Verification items for the finished model (mm, model axes). A direction names the side the tool comes from. Give positions to 0.01 mm unless a question says otherwise; leave off trailing zeros. Write each loop counter-clockwise with the first axis right and the second up, starting at its lowest first coordinate (ties: lowest second). Pieces come first, ordered by that corner, then holes. Notation, with made-up numbers: (84, 67) -> (131, 67) arc R26 ccw to (131, 100) -> close; hole circle Ø11 at (18, -14). An arc over 180 degrees is marked (long way). Use one line per item in the form item = value. Start each with the question number.
(1) Section check B-B, the plane x = 16.5. Record the cut outline in (y, z), plus the area to 3 significant figures.
(2) Set-up check for faces 1 (the face through (22, -11, 63.508)), 2 (the face through (21, 0, 34)): record each of +Z, -Z, +X, -X, +Y, -Y from which the full face is reachable in a straight line by a thin tool's end or side.
(3) Section check C-C, the plane y = -14.25. Record the cut outline in (x, z).
(4) Depth check by flat-ended pin: pin 1 Ø16.5 at (x, z) = (28.5, 30) entering from -Y; pin 2 Ø3.5 at (x, y) = (43.5, -12) entering from -Z; pin 3 Ø10.5 at (x, y) = (44.5, -13) entering from +Z. Enter the tip coordinate at first touch or a pass-through.
(5) Release check for a two-part mould opening along X. For faces 3 (the face through (53, -10, 32)), 4 (the face through (47, -10, 65)), 5 (the face through (0, -11, 61)) record: pulls with the +X half, pulls with the -X half, needs draft (parallel to the pull), parting line crosses it, or undercut.
(6) Section check A-A, the plane z = 59. Record the cut outline in (x, y), plus the area to 3 significant figures.
(7) Scan lines: L1, parallel to X at y = -9.5, z = 17.5; L2, parallel to Z at x = 3.5, y = -4.5; L3, parallel to Y at x = 24, z = 47. Record each from-to range of solid material in increasing order.
from build123d import *

# Parameters (mm, degrees)
F2_DEPTH  = 2
F0_W      = 4
F0_H      = 4
F0_H_2    = 57
F3_DEPTH  = 20
F3_FACE_W = 62.291004
F3_FACE_H = 20
F4_DEPTH  = 4.3
F5_DEPTH  = 4
F7_DEPTH  = 19.3


with BuildPart() as f2:
    # F0 (on Front) → F2 (new body)
    with BuildSketch(Plane.XZ):
        Polygon((-5.291004, 61), (-5.291004, 4), (0, 4), (49, 4), (49, 61), (37.840104, 61), (36.194602, 63.50845), (7.514394, 63.50845), (5.868892, 61), align=None)
    extrude(amount=F2_DEPTH)

    # F0 (on Front) → F3 (join)
    with BuildSketch(Plane.XZ):
        Polygon((-5.291004, 0), (0, 0), (53, 0), (53, 65), (40, 65), (38.354498, 67.50845), (5.354498, 67.50845), (3.708996, 65), (-5.291004, 65), (-5.291004, 61), (5.868892, 61), (7.514394, 63.50845), (36.194602, 63.50845), (37.840104, 61), (49, 61), (49, 4), (0, 4), (-5.291004, 4), align=None)
        with Locations((-7.291004, 2)):
            Rectangle(F0_W, F0_H)
        with Locations((-7.291004, 32.5)):
            Rectangle(F0_W, F0_H_2)
        with Locations((-7.291004, 63)):
            Rectangle(F0_W, F0_H)
    extrude(amount=F3_DEPTH)

    # F3_face (on face) → F4 (join)
    with BuildSketch(Plane(origin=(21.854498, -10, 0), x_dir=(1, 0, 0), z_dir=(0, 0, -1))):
        Rectangle(F3_FACE_W, F3_FACE_H)
    extrude(amount=-F4_DEPTH)

    # F3_face (on face) → F5 (join)
    with BuildSketch(Plane(origin=(21.854498, -10, 0), x_dir=(1, 0, 0), z_dir=(0, 0, -1))):
        Rectangle(F3_FACE_W, F3_FACE_H)
    extrude(amount=-F5_DEPTH)

    # F6 (on face) → F7 (cut)
    with BuildSketch(Plane.XZ.offset(20)):
        Polygon((49, 4.3), (-5.291004, 4.3), (-5.291004, 0), (49.075996, 0), (49.075996, 4.3), align=None)
    extrude(amount=-F7_DEPTH, mode=Mode.SUBTRACT)


solid = f2.part
Completed:
q1.outline = (-20, 63.51) -> (-2, 63.51) -> (-2, 4.3) -> (-0.7, 4.3) -> (-0.7, 0) -> (0, 0) -> (0, 67.51) -> (-20, 67.51) -> close
q1.area = 201 mm²
q2.face_1 = -Z, -Y
q2.face_2 = +Z, -Z, +X, -X, +Y
q3.outline = (-9.29, 0) -> (-5.29, 0) -> (-5.29, 61) -> (5.87, 61) -> (7.51, 63.51) -> (36.19, 63.51) -> (37.84, 61) -> (49, 61) -> (49, 4.3) -> (49.08, 4.3) -> (49.08, 0) -> (53, 0) -> (53, 65) -> (40, 65) -> (38.35, 67.51) -> (5.35, 67.51) -> (3.71, 65) -> (-9.29, 65) -> close
q4.pin_1 = -2
q4.pin_2 = 61
q4.pin_3 = 66.14
q5.face_3 = pulls with the +X half
q5.face_4 = needs draft
q5.face_5 = undercut
q6.outline = (-9.29, -20) -> (-5.29, -20) -> (-5.29, -2) -> (49, -2) -> (49, -20) -> (53, -20) -> (53, 0) -> (-9.29, 0) -> close
q6.area = 269 mm²
q7.L1 = -9.29 to -5.29, 49 to 53
q7.L2 = 61 to 65
q7.L3 = -2 to 0
